Verification items for this drawing (mm, ordinates from the low corner). A direction names the side the tool comes from. Round coordinates to 2 decimals unless told otherwise and drop trailing zeros. Order: outer loops, then holes, each group sorted by start corner. A loop starts at its lowest first (then second) coordinate and runs counter-clockwise, first axis right, second up. Notation, with made-up numbers: (75, 28) -> (86, 28) arc R27 cw to (86, 57) -> close; hole circle Ø7 at (36.25, 40). An arc over 180 degrees is marked (long way). Answer in a Markdown table with one row per item.
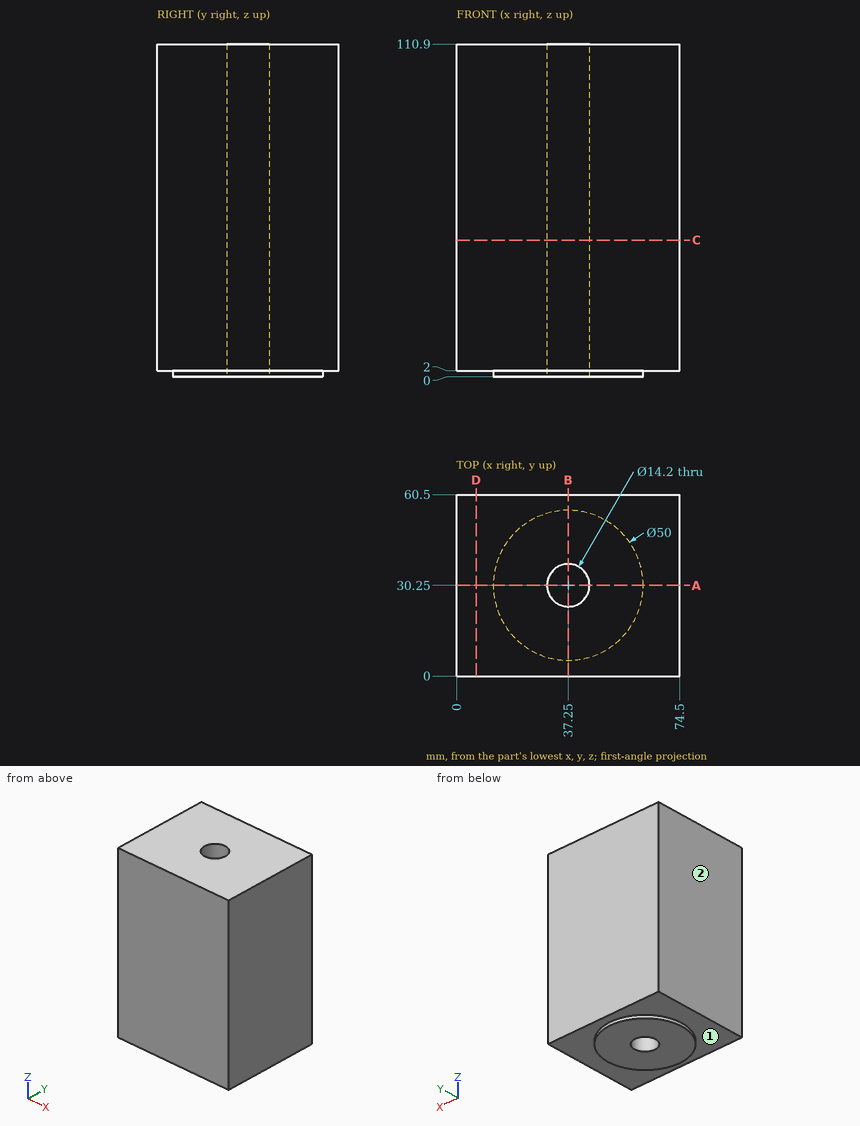
Item 1: Cross-section at A-A (y = 30.25). Record the boundary of the cut face in (x, z).
Result sheet:
| item | result |
|---|---|
| outline | (0, 2) -> (12.25, 2) -> (12.25, 0) -> (30.15, 0) -> (30.15, 110.9) -> (0, 110.9) -> close; (44.35, 0) -> (62.25, 0) -> (62.25, 2) -> (74.5, 2) -> (74.5, 110.9) -> (44.35, 110.9) -> close |
Item 2: Set-up check for the marked faces 1 and 2: record each of +Z, -Z, +X, -X, +Y, -Y from which the full face is reachable in a straight line by a thin tool's end or side.
Result sheet:
| item | result |
|---|---|
| face 1 | -Z |
| face 2 | +Z, -Z, -X, +Y, -Y |
Item 3: Cross-section at D-D (x = 6.5). Record the boundary of the cut face in (y, z).
Result sheet:
| item | result |
|---|---|
| outline | (0, 2) -> (60.5, 2) -> (60.5, 110.9) -> (0, 110.9) -> close |
Item 4: Cross-section at B-B (x = 37.25). Record the boundary of the cut face in (y, z).
Result sheet:
| item | result |
|---|---|
| outline | (0, 2) -> (5.25, 2) -> (5.25, 0) -> (23.15, 0) -> (23.15, 110.9) -> (0, 110.9) -> close; (37.35, 0) -> (55.25, 0) -> (55.25, 2) -> (60.5, 2) -> (60.5, 110.9) -> (37.35, 110.9) -> close |
Item 5: Depth check by flat-ended pin: P1, Ø11.5, axis at x = 37.25, y = 30.25, coming from the -Z side. Enter the tip coordinate at first touch or a pass-through.
Result sheet:
| item | result |
|---|---|
| P1 | passes through |
Item 6: Cross-section at C-C (z = 45.5). Record the boundary of the cut face in (x, y).
Result sheet:
| item | result |
|---|---|
| outline | (0, 0) -> (74.5, 0) -> (74.5, 60.5) -> (0, 60.5) -> close; hole circle Ø14.2 at (37.25, 30.25) |
Item 7: Scan lines: line 1 (Y direction, x = 37.25, z = 32.5); line 2 (Z direction, x = 25, y = 4); line 3 (X direction, y = 31.5, z = 11.5). Record each from-to range of solid material in increasing order. Write a range as [from, to].
Result sheet:
| item | result |
|---|---|
| line 1 | y = [0, 23.15], [37.35, 60.5] |
| line 2 | z = [2, 110.9] |
| line 3 | x = [0, 30.26], [44.24, 74.5] |
